Design review of the part built by this model. Coordinates are the model's own, in mm. A direction names the side the tool comes from. Round coordinates to 2 decimals unless told otherwise and drop trailing zeros. Write each loop counter-clockwise with the first axis right and the second up, starting at its lowest first coordinate (ties: lowest second). Pieces come first, ordered by that corner, then holes. Notation, with made-up numbers: M -38.75,63 L -17.75,63 A17 ccw -17.75,87 Z; hole C 71.25,31 d3. An arc over 180 degrees is marked long. Use CSV: the item, a comma, the result in double quotes.
from build123d import *

# Parameters (mm, degrees)
SKETCH_1_W          = 33.124171168
SKETCH_1_H          = 29.521848668
SKETCH_1_R          = 0.5
EXTRUDE_1_DEPTH     = 2
EXTRUDE_2_DEPTH     = 2
CUT_EXTRUDE_1_DEPTH = 6


with BuildPart() as part:
    # 草图1 → 凸台-拉伸1 (new body)
    with BuildSketch(Plane.XY):
        Rectangle(SKETCH_1_W, SKETCH_1_H)
        with Locations((0, 7.1)):
            Circle(SKETCH_1_R, mode=Mode.SUBTRACT)
        with Locations((7.1, 0)):
            Circle(SKETCH_1_R, mode=Mode.SUBTRACT)
        with Locations((0, -7.1)):
            Circle(SKETCH_1_R, mode=Mode.SUBTRACT)
        with Locations((-7.1, 0)):
            Circle(SKETCH_1_R, mode=Mode.SUBTRACT)
    extrude(amount=EXTRUDE_1_DEPTH)

    # 草图2 → 凸台-拉伸2 (add)
    with BuildSketch(Plane(origin=(16.562085584, 0, 0), x_dir=(0, 0, -1), z_dir=(1, 0, 0))):
        with BuildLine():
            Line((-5, -14.760924334), (0, -14.760924334))
            Line((0, -14.760924334), (0, 14.760924334))
            Line((0, 14.760924334), (-5, 14.760924334))
            ThreePointArc((-5, 14.760924334), (-7.828427125, 13.589351458), (-9, 10.760924334))
            Line((-9, 10.760924334), (-9, -10.760924334))
            ThreePointArc((-9, -10.760924334), (-7.828427125, -13.589351458), (-5, -14.760924334))
        make_face()
    extrude(amount=-EXTRUDE_2_DEPTH)

    # 草图3 → 切除-拉伸1 (cut)
    with BuildSketch(Plane(origin=(16.562085584, 0, 0), x_dir=(0, 0, -1), z_dir=(1, 0, 0))):
        with BuildLine():
            ThreePointArc((-7, -5), (-5.5, -6.5), (-4, -5))
            ThreePointArc((-4, -5), (-5.5, -3.5), (-7, -5))
        make_face()
        with BuildLine():
            ThreePointArc((-7, 5), (-5.5, 3.5), (-4, 5))
            ThreePointArc((-4, 5), (-5.5, 6.5), (-7, 5))
        make_face()
    extrude(amount=-CUT_EXTRUDE_1_DEPTH, mode=Mode.SUBTRACT)


solid = part.part
1) Add section A-A on y = -5. Write out the cut boundary in (x, z), then the cut area to 3 significant figures.
Answers:
outline,"M -16.56,0 L 16.56,0 L 16.56,4 L 14.56,4 L 14.56,2 L -16.56,2 Z; M 14.56,7 L 16.56,7 L 16.56,9 L 14.56,9 Z"
area,"74.2 mm²"
2) Add section C-C on x = 0. Write out the cut boundary in (y, z), then the cut area to 3 significant figures.
Answers:
outline,"M -14.76,0 L -7.6,0 L -7.6,2 L -14.76,2 Z; M -6.6,0 L 6.6,0 L 6.6,2 L -6.6,2 Z; M 7.6,0 L 14.76,0 L 14.76,2 L 7.6,2 Z"
area,"55.0 mm²"
3) Add section B-B on y = 0. Write out the cut boundary in (x, z).
Answers:
outline,"M -16.56,0 L -7.6,0 L -7.6,2 L -16.56,2 Z; M -6.6,0 L 6.6,0 L 6.6,2 L -6.6,2 Z; M 7.6,0 L 16.56,0 L 16.56,9 L 14.56,9 L 14.56,2 L 7.6,2 Z"
4) Machinability: for faces 1 (the face through (-1, 0, 2)), 2 (the face through (-0.108, 6.612, 0.986)), which of the approach directions +Z, -Z, +X, -X, +Y, -Y give a long, thin tool a straight path to every point of the face, cutting with its end or side? Answer none if there is none.
Answers:
face 1,"+Z, -X, +Y, -Y"
face 2,"+Z, -Z"
5) Add section D-D on z = 6. Write out the cut boundary in (x, y), then the cut area to 3 significant figures.
Answers:
outline,"M 14.56,-14.63 L 16.56,-14.63 L 16.56,-6.41 L 14.56,-6.41 Z; M 14.56,-3.59 L 16.56,-3.59 L 16.56,3.59 L 14.56,3.59 Z; M 14.56,6.41 L 16.56,6.41 L 16.56,14.63 L 14.56,14.63 Z"
area,"47.2 mm²"
6) For pin 1 Ø3 at (x, y) = (8, 10.5) entering from +Z; pin 2 Ø3 at (y, z) = (-2, 6.5) entering from -X, all flat-tipped, find the tip position at first contact; note any pin that passes through.
Answers:
pin 1,"z = 2"
pin 2,"x = 14.56"
7) The part is to be moulded in two halves that separate along X. For faces 3 (the face through (16, 0, 9)), 4 (the face through (6.6, 0, 1)), 5 (the face through (16.562, 0, 5)), say which applies: released by +X, released by -X, zero draft, split by the parting line, or undercut.
Answers:
face 3,"zero draft"
face 4,"undercut"
face 5,"released by +X"
8) Wall thickness on line 1 along Y through (x, z) = (0, 0.9); line 2 along Y through (x, z) = (-7.1, 1.65); line 3 along Y through (x, z) = (15.75, 5.5): over which ranges is each line inside the solid? List them lowest first. Write a range as [from, to].
Answers:
line 1,"[-14.76, -7.6], [-6.6, 6.6], [7.6, 14.76]"
line 2,"[-14.76, -0.5], [0.5, 14.76]"
line 3,"[-14.73, -6.5], [-3.5, 3.5], [6.5, 14.73]"
